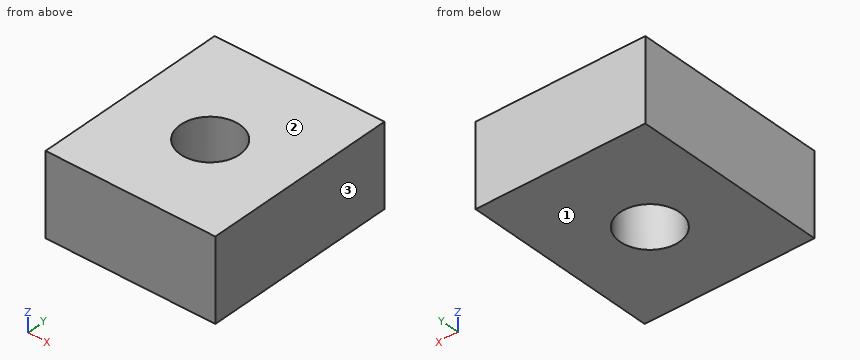
```python
from build123d import *

# Parameters (mm, degrees)
F0_W     = 65.93775
F0_H     = 31.747806
F1_DEPTH = 76.2
F2_R     = 11.490994
F3_DEPTH = 31.748807


with BuildPart() as f1:
    # F0 (on Front) → F1 (new body)
    with BuildSketch(Plane.XZ):
        Rectangle(F0_W, F0_H)
    extrude(amount=F1_DEPTH)

    # F2 (on face) → F3 (cut, through all)
    with BuildSketch(Plane.XY.offset(15.873903)):
        with Locations((0, -40.273719)):
            Circle(F2_R)
    extrude(amount=-F3_DEPTH, mode=Mode.SUBTRACT)


solid = f1.part
```
Here's how the part is built. I have some questions about the finished solid (model axes, mm). Face numbers are marked on the shaded views. Coordinates: 2 decimals unless noted, no trailing zeros. Write each loop counter-clockwise with the first axis right and the second up, starting at its lowest first coordinate (ties: lowest second). Pieces come first, ordered by that corner, then holes. Notation, with made-up numbers: (64.25, -33.75) -> (93.25, -33.75) arc R22 cw to (93.25, -9.75) -> close; hole circle Ø4 at (-1.5, 63). An arc over 180 degrees is marked (long way). Use a Markdown table: item, result. Add a question column.
(1) I'm going to push a flat-ended pin straight in: P1, Ø14, axis at x = 0, y = -40.27, coming from the -Z side. Where does the tip first touch, or does it pass through?
(2) If we section it at C-C, the plane z = -8: Write out the boundary of the cut face in (x, y).
(3) If we section it at B-B, the plane y = -33: Write out the boundary of the cut face in (x, z), and give its area (3 significant figures).
(4) If we section it at A-A, the plane x = 0: Write out the boundary of the cut face in (y, z), and give its area (3 significant figures).
(5) Please list where these lines run through material, in increasing order: line 1 (Y direction, x = 0, z = 2); line 2 (Y direction, x = -8, z = -10.5); line 3 (X direction, y = -39, z = 4.5).
(6) We'd pull the mould along Z, two halves only. Please class the marked faces 1, 2 and 3: +Z half, -Z half, draft (parallel to the pull), parting line (faces both ways), or undercut.
Outcome:
| question | item | result |
|---|---|---|
| 1 | P1 | passes through |
| 2 | outline | (-32.97, -76.2) -> (32.97, -76.2) -> (32.97, 0) -> (-32.97, 0) -> close; hole circle Ø22.98 at (0, -40.27) |
| 3 | outline | (-32.97, -15.87) -> (-8.9, -15.87) -> (-8.9, 15.87) -> (-32.97, 15.87) -> close; (8.9, -15.87) -> (32.97, -15.87) -> (32.97, 15.87) -> (8.9, 15.87) -> close |
| 3 | area | 1,530 mm^2 |
| 4 | outline | (-76.2, -15.87) -> (-51.76, -15.87) -> (-51.76, 15.87) -> (-76.2, 15.87) -> close; (-28.78, -15.87) -> (0, -15.87) -> (0, 15.87) -> (-28.78, 15.87) -> close |
| 4 | area | 1,690 mm^2 |
| 5 | line 1 | y = -76.2 to -51.76, -28.78 to 0 |
| 5 | line 2 | y = -76.2 to -48.52, -32.02 to 0 |
| 5 | line 3 | x = -32.97 to -11.42, 11.42 to 32.97 |
| 6 | face 1 | -Z half |
| 6 | face 2 | +Z half |
| 6 | face 3 | draft |
